Verification items for the finished model (mm, model axes). A direction names the side the tool comes from. Coordinates: 2 decimals unless noted, no trailing zeros. Loops run counter-clockwise (first coordinate to the right, second up) from the corner with the lowest first, then second, coordinate; pieces in that order, holes last. Notation, with made-up numbers: (-9, -36.5) - (40, -36.5) arc R22 cw to (40, 2.5) - close; hole circle Ø1 at (61.5, 59). An arc over 180 degrees is marked (long way). One line per item, written item: value. Start each with the question number.
(1) Thickness scan on probe 1 along Z at (x, y) = (1.75, 1.5); probe 2 along Z at (x, y) = (0.25, -5.5); probe 3 along Y at (x, z) = (1.25, 1.75). Record the ranges inside material, lowest first. Write a range as [from, to].
(2) Set-up check for faces 1 (the face through (-9, 0, 8)), 2 (the face through (-6.5, -5, 7)), 3 (the face through (0, -1, 6)), 4 (the face through (9, 0, 8)), 5 (the face through (0, -5, 3.5)): record each of +Z, -Z, +X, -X, +Y, -Y from which the full face is reachable in a straight line by a thin tool's end or side.
(3) Section check C-C (x = 5.5). Record the boundary of the cut face in (y, z), plus the area to 3 significant figures.
(4) Draft check along Z on faces 6 (the face through (-3.55, -0.93, 8.57)), 7 (the face through (-0.1, -6.25, 9.3)), 8 (the face through (-11, 0, 4.5)). Enter one of: +Z half, -Z half, draft (parallel to the pull), parting line (faces both ways), or undercut.
(5) Section check A-A (z = 8.5). Record the boundary of the cut face in (x, y).
(6) Gauge pin test, flat ends, axial feed: P1, Ø5, axis at x = 8.5, y = -2.5, coming from the -Z side; P2, Ø1.6, axis at y = -5, z = 6, coming from the -X side; P3, Ø2, axis at x = 12, y = 0, coming from the +Z side; P4, Ø1, axis at y = -3.5, z = 6, coming from the +X side. Record the tip position at first contact, or that the pin passes through.
```python
from build123d import *

# Parameters (mm, degrees)
F0_W     = 18
F0_H     = 7
F1_DEPTH = 4.25
F2_W     = 13
F2_H     = 8
F3_DEPTH = 2
F4_W     = 8
F4_H     = 3
F5_DEPTH = 10.5
F6_R     = 1.49999


# Not quite as in the source:
# - a fillet or chamfer is up to 0.001 mm smaller than in the source, because OpenCascade refuses the exact size


with BuildPart() as f1:
    # F0 (on Front) → F1 (new body, symmetric)
    with BuildSketch(Plane.XZ):
        Polygon((-13, 4.5), (-13, 0), (13, 0), (13, 4.5), (9, 4.5), (-9, 4.5), align=None)
        with Locations((0, 8)):
            Rectangle(F0_W, F0_H)
    extrude(amount=F1_DEPTH, both=True)

    # F2 (on face) → F3 (join)
    with BuildSketch(Plane.XZ.offset(4.25)):
        with Locations((0, 7.5)):
            Rectangle(F2_W, F2_H)
    extrude(amount=F3_DEPTH)

    # F4 (on face) → F5 (cut, through all)
    with BuildSketch(Plane.XZ.offset(6.25)):
        with Locations((0, 7.5)):
            Rectangle(F4_W, F4_H)
    extrude(amount=-F5_DEPTH, mode=Mode.SUBTRACT)

    # F6 (radius 1.5 in the source; OpenCascade refuses exactly that, so slightly less here)
    f6_edges = [f1.edges().sort_by_distance(p)[0] for p in [
        (-4, -1, 6),
        (-4, -1, 9),
        (4, -1, 6),
        (4, -1, 9),
    ]]
    fillet(f6_edges, radius=F6_R)


solid = f1.part
```
Responses:
1. probe 1: z = [0, 6], [9, 11.5]
1. probe 2: z = [3.5, 6], [9, 11.5]
1. probe 3: y = [-4.25, 4.25]
2. face 1: +Z, -X, +Y, -Y
2. face 2: +Z, -Z, -X, -Y
2. face 3: +Y, -Y
2. face 4: +Z, +X, +Y, -Y
2. face 5: -Z, +X, -X, -Y
3. outline: (-6.25, 3.5) - (-4.25, 3.5) - (-4.25, 0) - (4.25, 0) - (4.25, 11.5) - (-6.25, 11.5) - close
3. area: 114 mm²
4. face 6: undercut
4. face 7: draft
4. face 8: +Z half
5. outline: (-9, -4.25) - (-6.5, -4.25) - (-6.5, -6.25) - (-3.62, -6.25) - (-3.62, 4.25) - (-9, 4.25) - close; (3.62, -6.25) - (6.5, -6.25) - (6.5, -4.25) - (9, -4.25) - (9, 4.25) - (3.62, 4.25) - close
6. P1: stops at z = 0
6. P2: stops at x = -9
6. P3: stops at z = 4.5
6. P4: stops at x = 9
